```python
from build123d import *

# Parameters (mm, degrees)
BOSS_EXTRUDE1_DEPTH      = 15
BOSS_EXTRUDE1_DEPTH_BACK = 15
SKETCH1_W                = 30
SKETCH1_H                = 25
SKETCH2_R                = 12.7
CUT_EXTRUDE1_DEPTH       = 33.787192622


with BuildPart() as part:
    # Sketch1 → Boss-Extrude1 (new, two sides: drawn at the far end of the back side and taken through both)
    with BuildSketch(Plane(origin=(0, 0, 0), x_dir=(1, 0, 0), z_dir=(0, 1, 0)).offset(-BOSS_EXTRUDE1_DEPTH_BACK)):
        Rectangle(SKETCH1_W, SKETCH1_H)
    extrude(amount=BOSS_EXTRUDE1_DEPTH + BOSS_EXTRUDE1_DEPTH_BACK)

    # Sketch2 → Cut-Extrude1 (cut, through all)
    with BuildSketch(Plane.XY.offset(12.5)):
        Circle(SKETCH2_R)
    extrude(amount=-CUT_EXTRUDE1_DEPTH, mode=Mode.SUBTRACT)


solid = part.part
```
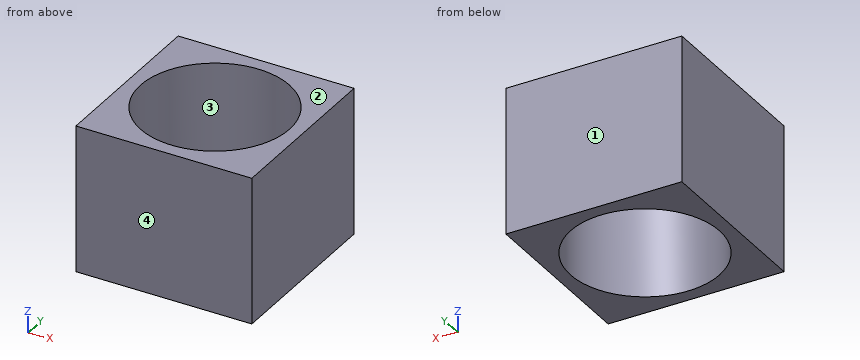
For this review, take the finished solid that the model builds, in its own axes (mm). Face numbers are marked on the shaded views. Round coordinates to 2 decimals unless told otherwise and drop trailing zeros. Write each loop counter-clockwise with the first axis right and the second up, starting at its lowest first coordinate (ties: lowest second). Pieces come first, ordered by that corner, then holes.
1) For line 1 along Y through (x, z) = (0, 1); line 2 along Y through (x, z) = (3.5, 9.75); line 3 along X through (y, z) = (10, -0.5), list the stretches that pass through material, from the lowest coordinate up.
Answer below:
line 1: y = -15 to -12.7, 12.7 to 15
line 2: y = -15 to -12.21, 12.21 to 15
line 3: x = -15 to -7.83, 7.83 to 15
2) Take a section at C-C on z = 5.75. Give the boundary of the cut face in (x, y), then the cut area to 3 significant figures.
Answer below:
outline: (-15, -15) - (15, -15) - (15, 15) - (-15, 15) - close; hole circle Ø25.4 at (0, 0)
area: 393 mm2
3) Mouldability with a two-part tool opening along Y and no side actions: class the marked faces 1, 2, 3 and 4 as +Y half, -Y half, draft (parallel to the pull), parting line (faces both ways), or undercut.
Answer below:
face 1: +Y half
face 2: draft
face 3: undercut
face 4: -Y half
4) Take a section at A-A on y = 0. Give the boundary of the cut face in (x, z).
Answer below:
outline: (-15, -12.5) - (-12.7, -12.5) - (-12.7, 12.5) - (-15, 12.5) - close; (12.7, -12.5) - (15, -12.5) - (15, 12.5) - (12.7, 12.5) - close
5) Insertion check: pin 1 Ø2 at (x, y) = (10, 4) entering from -Z. The pin has a flat end and moves straight along its axis. Give the tip position at first contact, or say it passes through.
Answer below:
pin 1: passes through
